Drawing for the job (mm, zero at the part's lowest x, y, z). A direction names the side the tool comes from. Give positions to 0.01 mm unless a question says otherwise; leave off trailing zeros. Write each loop counter-clockwise with the first axis right and the second up, starting at its lowest first coordinate (ties: lowest second). Pieces come first, ordered by that corner, then holes. Notation, with made-up numbers: (6, 26) - (21, 26) arc R13 cw to (21, 35) - close; hole circle Ø4 at (66.5, -10.5). An arc over 180 degrees is marked (long way). Answer as a JSON object with one key per item and string values. Group by question number.
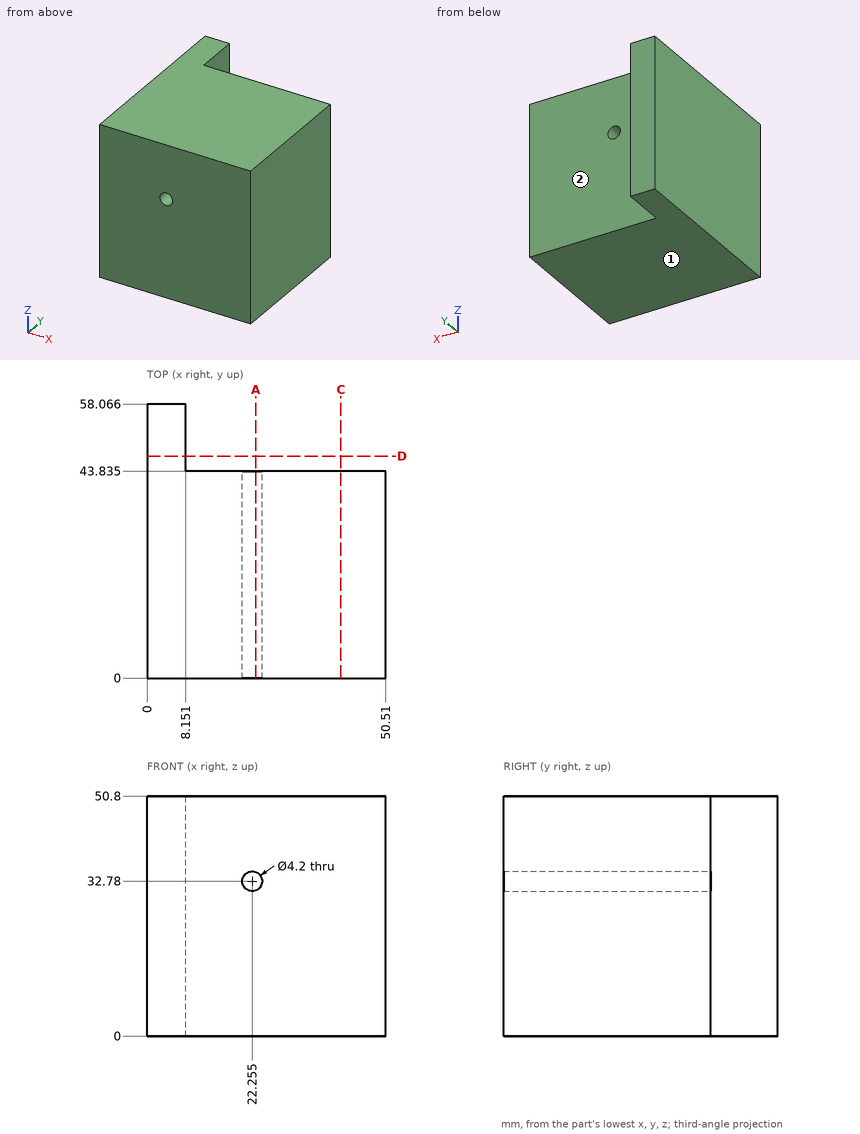
1) Band-saw the part on C-C (x = 41). List the corners of the cut face in (y, z) (1 decimal), plus the area to 3 significant figures.
2) Band-saw the part on A-A (x = 23). List the corners of the cut face in (y, z) (1 decimal), plus the area to 3 significant figures.
3) Drop flat-ended pins along their axis: P1, Ø1.5, axis at x = 29.5, z = 11.5, coming from the +Y side (1 decimal); P2, Ø15.5, axis at y = 54.5, z = 13, coming from the +X side. Give the stop position or say it passes through.
4) Band-saw the part on D-D (y = 47). List the corners of the cut face in (x, z), plus the area to 3 significant figures.
5) Probe line 1 (Y direction, x = 21, z = 42) (1 decimal); line 2 (X direction, y = 48, z = 46); line 3 (X direction, y = 17, z = 31) (1 decimal). List the from-to ranges inside material, lowest first.
6) Which spindle directions (+Z, -Z, +X, -X, +Y, -Y) get a long thin tool onto all of the face, cutting with end or side? Do the marked faces 1 and 2. Say none if no direction does.
Verdict:
{
 "1": {"outline": "(0, 0) - (43.8, 0) - (43.8, 50.8) - (0, 50.8) - close", "area": "2,230 mm2"},
 "2": {"outline": "(0, 0) - (43.8, 0) - (43.8, 30.8) - (0, 30.8) - close; (0, 34.7) - (43.8, 34.7) - (43.8, 50.8) - (0, 50.8) - close", "area": "2,050 mm2"},
 "3": {"P1": "y = 43.8", "P2": "x = 8.15"},
 "4": {"outline": "(0, 0) - (8.15, 0) - (8.15, 50.8) - (0, 50.8) - close", "area": "414 mm2"},
 "5": {"line 1": "0 to 43.8", "line 2": "0 to 8.15", "line 3": "0 to 21.1, 23.4 to 50.5"},
 "6": {"face 1": "-Z, +X, -X, +Y, -Y", "face 2": "+Z, -Z, +X, +Y"}
}
